from build123d import *

# Parameters (mm, degrees)
FLOWER_R       = 4
FLOWER_R_2     = 1.885
MOUNTING_DEPTH = 99.604197228


with BuildPart() as part:
    # Wheel Arc → Wheel (revolve)
    with BuildSketch(Plane.XY, mode=Mode.PRIVATE) as wheel_sk:
        with BuildLine():
            Line((-25.4, 0), (25.4, 0))
            Line((25.4, 0), (25.4, -58.170962527))
            ThreePointArc((25.4, -58.170962527), (24.634795193, -59.528897306), (23.076866942, -59.577731965))
            ThreePointArc((23.076866942, -59.577731965), (17.93994263, -57.251785424), (12.573, -55.521483285))
            Line((12.573, -55.521483285), (12.573, -52.9082))
            Line((12.573, -52.9082), (-12.573, -52.9082))
            Line((-12.573, -52.9082), (-12.573, -55.521483285))
            ThreePointArc((-12.573, -55.521483285), (-17.93994263, -57.251785424), (-23.076866942, -59.577731965))
            ThreePointArc((-23.076866942, -59.577731965), (-24.634795193, -59.528897306), (-25.4, -58.170962527))
            Line((-25.4, -58.170962527), (-25.4, 0))
        make_face()
    revolve(wheel_sk.sketch.rotate(Axis((-40.905271883, 0, 0), (1, 0, 0)), 270), axis=Axis((-40.905271883, 0, 0), (1, 0, 0)))

    # Flower → Mounting (cut, through all)
    with BuildSketch(Plane(origin=(25.4, 0, 0), x_dir=(0, 0, -1), z_dir=(1, 0, 0))):
        Circle(FLOWER_R)
        with Locations((0, 8)):
            Circle(FLOWER_R_2)
        with Locations((8, 0)):
            Circle(FLOWER_R_2)
        with Locations((0, -8)):
            Circle(FLOWER_R_2)
        with Locations((-8, 0)):
            Circle(FLOWER_R_2)
    extrude(amount=-MOUNTING_DEPTH, mode=Mode.SUBTRACT)


solid = part.part
For this review, take the finished solid that the model builds, in its own axes (mm). A direction names the side the tool comes from. Coordinates: 2 decimals unless noted, no trailing zeros. Loops run counter-clockwise (first coordinate to the right, second up) from the corner with the lowest first, then second, coordinate; pieces in that order, holes last. Notation, with made-up numbers: (4, 51) - (33, 51) arc R31 ccw to (33, 87) - close; hole circle Ø6 at (58.25, -7). An arc over 180 degrees is marked (long way). Use a Markdown table: item, result. Add a question column.
Item 1: Tool access review of faces 1 (the face through (-12.573, 20.3, -49.1)), 2 (the face through (0.36, 6.16, 0.41)): name each direction out of +Z, -Z, +X, -X, +Y, -Y from which nothing blocks a thin tool from reaching the whole face with its end or side.
Item 2: For line 1 (Y direction, x = 11, z = 0) (3 decimals); line 2 (Z direction, x = -10, y = 2); line 3 (Z direction, x = -20.5, y = 8.5), list the stretches that pass through material, from the lowest coordinate up.
Item 3: We need section B-B (x = -11). Give the boundary of the cut face in (y, z) (3 decimals).
Item 4: We need section A-A (z = 0). Give the boundary of the cut face in (x, y) (1 decimal), and give its area (3 significant figures).
Item 5: Mouldability with a two-part tool opening along Y and no side actions: class faces 3 (the face through (0.356, 0.083, 9.883)), 4 (the face through (-0.176, -15.892, 50.465)), 5 (the face through (12.573, 20.3, 49.1)), 6 (the face through (0.356, -3.905, 0.867)) as pulls with the +Y half, pulls with the -Y half, needs draft (parallel to the pull), parting line crosses it, or undercut.
Item 6: Insertion check: pin 1 Ø12 at (x, y) = (9, 42.5) entering from -Z; pin 2 Ø4.5 at (y, z) = (0, -8) entering from +X; pin 3 Ø1 at (x, z) = (14.5, 46) entering from -Y; pin 4 Ø1 at (x, y) = (-5.5, 43) entering from +Z. Each pin has a flat end and moves straight along its axis. Give the tip position at first contact, or say it passes through.
Results list:
| question | item | result |
|---|---|---|
| 1 | face 1 | none |
| 1 | face 2 | +X, -X |
| 2 | line 1 | y = -52.908 to -9.885, -6.115 to -4, 4 to 6.115, 9.885 to 52.908 |
| 2 | line 2 | z = -52.87 to -3.46, 3.46 to 52.87 |
| 2 | line 3 | z = -57.7 to -1.82, 1.82 to 57.7 |
| 3 | outline | circle Ø105.816 at (0, 0); hole circle Ø3.77 at (-8, 0); hole circle Ø8 at (0, 0); hole circle Ø3.77 at (0, -8); hole circle Ø3.77 at (0, 8); hole circle Ø3.77 at (8, 0) |
| 4 | outline | (-25.4, -58.2) arc R1.6 ccw to (-23.1, -59.6) arc R49.8 cw to (-12.6, -55.5) - (-12.6, -52.9) - (12.6, -52.9) - (12.6, -55.5) arc R49.8 cw to (23.1, -59.6) arc R1.6 ccw to (25.4, -58.2) - (25.4, -9.9) - (-25.4, -9.9) - close; (-25.4, -6.1) - (25.4, -6.1) - (25.4, -4) - (-25.4, -4) - close; (-25.4, 4) - (25.4, 4) - (25.4, 6.1) - (-25.4, 6.1) - close; (-25.4, 9.9) - (25.4, 9.9) - (25.4, 58.2) arc R1.6 ccw to (23.1, 59.6) arc R49.8 cw to (12.6, 55.5) - (12.6, 52.9) - (-12.6, 52.9) - (-12.6, 55.5) arc R49.8 cw to (-23.1, 59.6) arc R1.6 ccw to (-25.4, 58.2) - close |
| 4 | area | 4,830 mm^2 |
| 5 | face 3 | undercut |
| 5 | face 4 | parting line crosses it |
| 5 | face 5 | needs draft |
| 5 | face 6 | undercut |
| 6 | pin 1 | stops at z = -40.78 |
| 6 | pin 2 | stops at x = 25.4 |
| 6 | pin 3 | stops at y = -32.81 |
| 6 | pin 4 | stops at z = 31.51 |
